```python
from build123d import *

# Parameters (mm, degrees)
SKETCH_R        = 13.5
SKETCH_R_2      = 6.75
PAD_DEPTH       = 1
SKETCH001_R     = 13.5
PAD001_DEPTH    = 1
SKETCH002_R     = 6.75
PAD002_DEPTH    = 25
POCKET_DEPTH    = 30
FILLET_R        = 1
SKETCH004_R     = 13.5
PAD003_DEPTH    = 2
CHAMFER_SIZE    = 1
CHAMFER001_SIZE = 0.5
CHAMFER002_SIZE = 0.5


with BuildPart() as part:
    # Sketch → Pad (new body)
    with BuildSketch(Plane.XY):
        Circle(SKETCH_R)
        Circle(SKETCH_R_2, mode=Mode.SUBTRACT)
    extrude(amount=-PAD_DEPTH)

    # Sketch001 → Pad001 (join)
    with BuildSketch(Plane.XY):
        Circle(SKETCH001_R)
    extrude(amount=PAD001_DEPTH)

    # Sketch002 → Pad002 (join)
    with BuildSketch(Plane.XY):
        Circle(SKETCH002_R)
    extrude(amount=PAD002_DEPTH)

    # Sketch003 → Pocket (cut)
    with BuildSketch(Plane.XY):
        Polygon((-5.629165, 3.25), (5.629165, 3.25), (0, -6.5), align=None)
    extrude(amount=POCKET_DEPTH, mode=Mode.SUBTRACT)

    # Fillet
    fillet_edges = [part.edges().sort_by_distance(p)[0] for p in [
        (5.629165, 3.25, 12.5),
        (-5.629165, 3.25, 12.5),
        (0, -6.5, 12.5),
    ]]
    fillet(fillet_edges, radius=FILLET_R)

    # Sketch004 (on DatumPlane) → Pad003 (join)
    with BuildSketch(Plane.XY.offset(25)):
        Circle(SKETCH004_R)
    extrude(amount=PAD003_DEPTH)

    # Chamfer
    chamfer_edges = [part.edges().sort_by_distance(p)[0] for p in [
        (-6.75, 0, 1),
        (-6.75, 0, 25),
    ]]
    chamfer(chamfer_edges, length=CHAMFER_SIZE)

    # Chamfer001
    chamfer001_edges = [part.edges().sort_by_distance(p)[0] for p in [
        (-6.75, 0, -1),
    ]]
    chamfer(chamfer001_edges, length=CHAMFER001_SIZE)

    # Chamfer002
    chamfer002_edges = [part.edges().sort_by_distance(p)[0] for p in [
        (2.814583, -1.625, 0),
    ]]
    chamfer(chamfer002_edges, length=CHAMFER002_SIZE)


solid = part.part
```
Here's how the part is built. I have some questions about the finished solid (model axes, mm). A direction names the side the tool comes from. Coordinates: 2 decimals unless noted, no trailing zeros. Write each loop counter-clockwise with the first axis right and the second up, starting at its lowest first coordinate (ties: lowest second). Pieces come first, ordered by that corner, then holes. Notation, with made-up numbers: (85.25, -36) -> (127.25, -36) arc R24 ccw to (127.25, -4) -> close; hole circle Ø8 at (23, -2). An arc over 180 degrees is marked (long way). Use a Markdown table: item, result. Add a question column.
(1) If we section it at C-C, the plane x = 0: Write out the boundary of the cut face in (y, z).
(2) We'd pull the mould along Y, two halves only. Please class faces 4 (the cylindrical face through (-2.93, -13.18, 25.99)), 5 (the flat face through (2.84, -1.58, 12.58)): +Y half, -Y half, draft (parallel to the pull), parting line (faces both ways), or undercut.
(3) If we section it at B-B, the plane z = 15: Write out the boundary of the cut face in (x, y).
(4) If we section it at D-D, the plane x = 10.75: Write out the boundary of the cut face in (y, z), and give its area (3 significant figures).
(5) For faces 1 (the cylindrical face through (-2.93, -13.18, 0.01)), 2 (the flat face through (-3, -1.8, 0.25)), 3 (the cylindrical face through (-1.46, -6.59, 12.85)), which set-ups out of +Z, -Z, +X, -X, +Y, -Y let a thin tool reach every point of the face, with its end or its side?
(6) If we section it at A-A, the plane y = 11.5: Write out the boundary of the cut face in (x, z).
(7) I'm going to push flat-ended pins straight in: P1, Ø6, axis at y = -4.5, z = 19.5, coming from the -X side; P2, Ø2.5, axis at x = 1.5, z = 15, coming from the -Y side; P3, Ø13.5, axis at x = 0.5, y = -1.5, coming from the -Z side; P4, Ø2, axis at x = 0, z = 22.5, coming from the +Y side. Where does each tip first touch, or does it pass through?
(8) Please list where these lines run through material, in increasing order: line 1 (Y direction, x = 0, z = -0.35); line 2 (Z direction, x = 4, y = -11); line 3 (X direction, y = -3.5, z = 4.25).
Outcome:
| question | item | result |
|---|---|---|
| 1 | outline | (-13.5, -1) -> (-7.25, -1) -> (-6.75, -0.5) -> (-6.75, 0) -> (-6, 0) -> (-5.5, 0.5) -> (-5.5, 25) -> (3.25, 25) -> (3.25, 0.5) -> (3.75, 0) -> (6.75, 0) -> (6.75, -0.5) -> (7.25, -1) -> (13.5, -1) -> (13.5, 1) -> (7.75, 1) -> (6.75, 2) -> (6.75, 24) -> (7.75, 25) -> (13.5, 25) -> (13.5, 27) -> (-13.5, 27) -> (-13.5, 25) -> (-7.75, 25) -> (-6.75, 24) -> (-6.75, 2) -> (-7.75, 1) -> (-13.5, 1) -> close |
| 2 | face 4 | parting line |
| 2 | face 5 | undercut |
| 3 | outline | circle Ø13.5 at (0, 0); hole (-4.76, 1.75) -> (-0.87, -5) arc R1 ccw to (0.87, -5) -> (4.76, 1.75) arc R1 ccw to (3.9, 3.25) -> (-3.9, 3.25) arc R1 ccw to start |
| 4 | outline | (-8.17, -1) -> (8.17, -1) -> (8.17, 1) -> (-8.17, 1) -> close; (-8.17, 25) -> (8.17, 25) -> (8.17, 27) -> (-8.17, 27) -> close |
| 4 | area | 65.3 mm^2 |
| 5 | face 1 | +Z, -Z |
| 5 | face 2 | -Z |
| 5 | face 3 | none |
| 6 | outline | (-7.07, -1) -> (7.07, -1) -> (7.07, 1) -> (-7.07, 1) -> close; (-7.07, 25) -> (7.07, 25) -> (7.07, 27) -> (-7.07, 27) -> close |
| 7 | P1 | stops at x = -6.58 |
| 7 | P2 | stops at y = -6.75 |
| 7 | P3 | stops at z = -1 |
| 7 | P4 | stops at y = 6.75 |
| 8 | line 1 | y = -13.5 to -6.75, 6.75 to 13.5 |
| 8 | line 2 | z = -1 to 1, 25 to 27 |
| 8 | line 3 | x = -5.77 to -1.73, 1.73 to 5.77 |
